from build123d import *

# Parameters (mm, degrees)
F1_DEPTH  = 50
F3_DEPTH  = 9
F4_R      = 5
F5_DEPTH  = 100
F7_DEPTH  = 8
F9_DEPTH  = 42
F11_DEPTH = 13
F12_W     = 5.5079008639
F12_H     = 3.6583239734
F13_DEPTH = 25
F15_DEPTH = 5
F16_R     = 5
F17_DEPTH = 8
F19_DEPTH = 70.001
F20_W     = 50
F20_H     = 12
F21_DEPTH = 63.001
F22_R     = 5
F23_DEPTH = 63.001
F25_DEPTH = 50.001


with BuildPart() as f1:
    # F0 (on Front) → F1 (new body)
    with BuildSketch(Plane.XZ):
        Polygon((-50, 31.5), (-50, -31.5), (50, -31.5), (50, 16.5), (10, 16.5), (10, 31.5), align=None)
    extrude(amount=F1_DEPTH)

    # F2 (on face) → F3 (cut)
    with BuildSketch(Plane.XZ.offset(50)):
        with BuildLine():
            ThreePointArc((50, -16.5), (64.1421356237, -10.6421356237), (70, 3.5))
            ThreePointArc((70, 3.5), (50, 23.5), (30, 3.5))
            ThreePointArc((30, 3.5), (35.8578643763, -10.6421356237), (50, -16.5))
        make_face()
        with BuildLine():
            Line((30, 16.5), (30, 3.5))
            ThreePointArc((30, 3.5), (31.2386876382, 10.4291527956), (34.8013158464, 16.5))
            Line((34.8013158464, 16.5), (30, 16.5))
        make_face()
    extrude(amount=-F3_DEPTH, mode=Mode.SUBTRACT)

    # F4 (on face) → F5 (cut)
    with BuildSketch(Plane.XZ.offset(41)):
        with Locations((40, 5.378967151)):
            Circle(F4_R)
    extrude(amount=-F5_DEPTH, mode=Mode.SUBTRACT)

    # F6 (on face) → F7 (cut)
    with BuildSketch(Plane.XZ.offset(50)):
        with BuildLine():
            ThreePointArc((-50, -21.5), (-32.3223304703, -14.1776695297), (-25, 3.5))
            ThreePointArc((-25, 3.5), (-67.6776695297, 21.1776695297), (-50, -21.5))
        make_face()
        with BuildLine():
            Line((-50, 31.5), (-50, 28.5))
            ThreePointArc((-50, 28.5), (-32.3223304703, 21.1776695297), (-25, 3.5))
            Line((-25, 3.5), (-25, 31.5))
            Line((-25, 31.5), (-50, 31.5))
        make_face()
    extrude(amount=-F7_DEPTH, mode=Mode.SUBTRACT)

    # F8 (on face) → F9 (cut)
    with BuildSketch(Plane(origin=(0, 0, 0), x_dir=(-1, 0, 0), z_dir=(0, 1, 0))):
        with BuildLine():
            ThreePointArc((50, -26.5), (71.2132034356, -17.7132034356), (80, 3.5))
            ThreePointArc((80, 3.5), (50, 33.5), (20, 3.5))
            ThreePointArc((20, 3.5), (28.7867965644, -17.7132034356), (50, -26.5))
        make_face()
        with BuildLine():
            Line((20, 31.5), (20, 3.5))
            ThreePointArc((20, 3.5), (25.2703630392, 20.4836702684), (39.2296703857, 31.5))
            Line((39.2296703857, 31.5), (20, 31.5))
        make_face()
    extrude(amount=-F9_DEPTH, mode=Mode.SUBTRACT)

    # F10 (on face) → F11 (cut)
    with BuildSketch(Plane.XZ.offset(50)):
        with BuildLine():
            ThreePointArc((-20, -21.5), (-2.3223304703, -14.1776695297), (5, 3.5))
            ThreePointArc((5, 3.5), (-37.6776695297, 21.1776695297), (-20, -21.5))
        make_face()
    extrude(amount=-F11_DEPTH, mode=Mode.SUBTRACT)

    # F12 (on face) → F13 (cut)
    with BuildSketch(Plane(origin=(0, -42, 0), x_dir=(-1, 0, 0), z_dir=(0, 1, 0))):
        with Locations((22.7539504319, 29.6708380133)):
            Rectangle(F12_W, F12_H)
    extrude(amount=-F13_DEPTH, mode=Mode.SUBTRACT)

    # F14 (on face) → F15 (join)
    with BuildSketch(Plane.XZ.offset(37)):
        with BuildLine():
            ThreePointArc((-20, 3.5), (-20.4196010845, -1.5), (-21.6666666667, -6.3601329718))
            ThreePointArc((-21.6666666667, -6.3601329718), (-10.0350281055, 2.6637373972), (-20, 13.5))
            Line((-20, 13.5), (-20, 3.5))
        make_face()
    extrude(amount=F15_DEPTH)

    # F16 (on face) → F17 (join)
    with BuildSketch(Plane.XZ.offset(42)):
        with Locations((-20, 3.5)):
            Circle(F16_R)
    extrude(amount=F17_DEPTH)

    # F18 (on face) → F19 (cut, through all)
    with BuildSketch(Plane(origin=(-20, 0, 0), x_dir=(0, -1, 0), z_dir=(-1, 0, 0))):
        Polygon((0, 31.5), (0, 13.5), (6.5514642168, 31.5), align=None)
    extrude(amount=-F19_DEPTH, mode=Mode.SUBTRACT)

    # F20 (on face) → F21 (cut, through all)
    with BuildSketch(Plane.XY.offset(31.5)):
        with Locations((25, -6)):
            Rectangle(F20_W, F20_H)
    extrude(amount=-F21_DEPTH, mode=Mode.SUBTRACT)

    # F22 (on face) → F23 (cut, through all)
    with BuildSketch(Plane.XY.offset(31.5)):
        with Locations((-11, -20)):
            Circle(F22_R)
    extrude(amount=-F23_DEPTH, mode=Mode.SUBTRACT)

    # F24 (on face) → F25 (cut, through all)
    with BuildSketch(Plane.XZ.offset(50)):
        with BuildLine():
            Line((22.3409673765, -25.2284990706), (-5, -31.5))
            Line((-5, -31.5), (35, -31.5))
            Line((35, -31.5), (31.4479835543, -27.9479835543))
            ThreePointArc((31.4479835543, -27.9479835543), (27.2382101912, -25.437141636), (22.3409673765, -25.2284990706))
        make_face()
    extrude(amount=-F25_DEPTH, mode=Mode.SUBTRACT)


solid = f1.part
Can you work these out from the model? Positions are in its coordinate system, mm. A direction names the side the tool comes from. Coordinates: 2 decimals unless noted, no trailing zeros. Loops run counter-clockwise (first coordinate to the right, second up) from the corner with the lowest first, then second, coordinate; pieces in that order, holes last. Notation, with made-up numbers: M 29.25,-14.75 L 85.25,-14.75 A20 cw 85.25,19.25 Z; hole C 9.5,3 d9. An arc over 180 degrees is marked long. Return JSON: item names as keys, results as strings. Group by question number.
Item 1: Imagine slicing it at C-C (y = -20). Please give me the cut outline in (x, z), and give its area (3 significant figures).
Item 2: Thinking about a two-plate mould opening in Z: for faces 6 (the cylindrical face through (-24.995, -45.944, 3.72)), 7 (the cylindrical face through (35.005, -26.703, 5.599)), 8 (the flat face through (30, -31, 16.5)), 9 (the flat face through (-40, -42, -23)), which applies, released by +Z, released by -Z, zero draft, split by the parting line, or undercut?
Item 3: I'm going to push flat-ended pins straight in: pin 1 Ø2 at (x, y) = (8.5, -9.5) entering from +Z; pin 2 Ø4 at (x, y) = (34.5, -44) entering from +Z; pin 3 Ø22.5 at (y, z) = (-36, 12) entering from -X; pin 4 Ø11 at (x, z) = (-39, -23) entering from +Y. Where does each tip first touch, or does it pass through?
Item 4: If I drill on L1, parallel to Z at x = 40, y = -19; L2, parallel to X at y = -17, z = 5; L3, parallel to X at y = -19, z = 3, over which ranges is the centre line in solid material (lowest first)? Write a range as from..to.
Item 5: Imagine slicing it at B-B (x = 40). Please give me the cut outline in (y, z).
Item 6: Imagine slicing it at A-A (z = -4). Please give me the cut outline in (x, y), and give its area (3 significant figures).
Item 7: Imagine slicing it at D-D (z = 27). Please give me the cut outline in (x, y), and give its area (3 significant figures).
Item 8: On a 3-axis mill with a long thin cutter (end or side, diameter ignored), from which of +Z, -Z, +X, -X, +Y, -Y can I reach the whole of each face in a straight line? I mean faces 1 (the flat face through (0, -6, 1)), 2 (the flat face through (-22, -42, 4)), 3 (the flat face through (-9, -37, -2)), 4 (the flat face through (30, -46, 10)), 5 (the flat face through (10, -31, 24)). Say none if no direction works.
Verdict:
{
 "1": {"outline": "M -50,-31.5 L -16,-31.5 L -16,31.5 L -20,31.5 L -20,3.5 A30 cw -50,-26.5 Z; M -6,-31.5 L -5,-31.5 L 22.34,-25.23 A10 cw 31.45,-27.95 L 35,-31.5 L 50,-31.5 L 50,16.5 L 10,16.5 L 10,31.5 L -6,31.5 Z; hole C 40,5.38 d10", "area": "3,300 mm^2"},
 "2": {"face 6": "undercut", "face 7": "undercut", "face 8": "released by +Z", "face 9": "zero draft"},
 "3": {"pin 1": "passes through", "pin 2": "stops at z = -6.18", "pin 3": "stops at x = -25", "pin 4": "stops at y = 0"},
 "4": {"L1": "z = -31.5..0.38, 10.38..16.5", "L2": "x = -20..-15, -7..35.01, 44.99..50", "L3": "x = -20..-15.9, -6.1..35.6, 44.4..50"},
 "5": {"outline": "M -50,-31.5 L -12,-31.5 L -12,0.38 L -41,0.38 L -41,-13.82 L -50,-13.82 Z; M -41,10.38 L -12,10.38 L -12,16.5 L -41,16.5 Z"},
 "6": {"outline": "M -20.95,-42 L -13.39,-42 L -13.39,-37 L 3.85,-37 L 3.85,-50 L 31.46,-50 L 31.46,-41 L 50,-41 L 50,-12 L 0,-12 L 0,0 L -20.95,0 Z; hole C -11,-20 d10", "area": "2,420 mm^2"},
 "7": {"outline": "M -20,-37 L -11.47,-37 L -11.47,-50 L 10,-50 L 10,-12 L 0,-12 L 0,-4.91 L -20,-4.91 Z; hole C -11,-20 d10", "area": "1,090 mm^2"},
 "8": {"face 1": "+Z, -Z, +X, +Y", "face 2": "+Z, -X, +Y", "face 3": "-Y", "face 4": "+Z, +X, -Y", "face 5": "+Z, +X, +Y, -Y"}
}
